Could you check a few things on this drawing? It's one solid part, dimensions in mm from its lowest x, y, z. A direction names the side the tool comes from. Give positions to 0.01 mm unless a question says otherwise; leave off trailing zeros. Write each loop counter-clockwise with the first axis right and the second up, starting at its lowest first coordinate (ties: lowest second). Pieces come first, ordered by that corner, then holes.
1. Suppose I cut it at B-B (y = 170). Please give me the cut outline in (x, z).
2. If I drill on probe 1 along Y at (x, z) = (35, 1.15); probe 2 along Z at (x, y) = (31, 127.5); probe 3 along Y at (x, z) = (13, 27), over which ranges is the centre line in solid material (lowest first)?
3. Suppose I cut it at A-A (x = 35). Please give me the cut outline in (y, z).
4. Thinking about a two-plate mould opening in Z: for the marked faces 4, 5 and 6, which applies, pulls with the +Z half, pulls with the -Z half, needs draft (parallel to the pull), parting line crosses it, or undercut?
5. I'm going to push flat-ended pins straight in: pin 1 (4 mm diameter, centred on x = 69, y = 89.5, fed in from -Z); pin 2 (12.5 mm diameter, centred on x = 31, z = 20.5, fed in from +Y); pin 3 (20 mm diameter, centred on x = 35, y = 170, fed in from +Z). Where does each tip first touch, or does it pass through?
6. Suppose I cut it at D-D (y = 15). Please give me the cut outline in (x, z), and give its area (3 significant figures).
7. Suppose I cut it at C-C (x = 20.5). Please give me the cut outline in (y, z).
8. On a 3-axis mill with a long thin cutter (end or side, diameter ignored), from which of +Z, -Z, +X, -X, +Y, -Y can I reach the whole of each face in a straight line? I mean the marked faces 1, 2 and 3. Say none if no direction works.
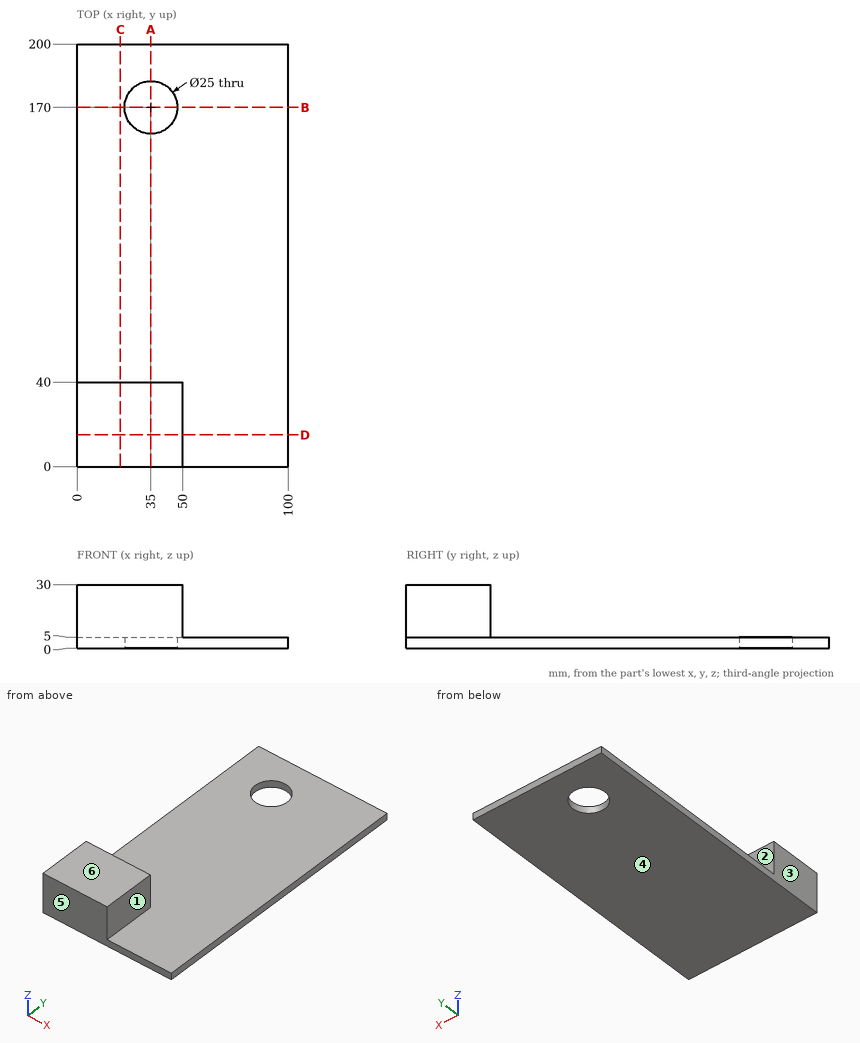
Checks:
1. outline: (0, 0) - (22.5, 0) - (22.5, 5) - (0, 5) - close; (47.5, 0) - (100, 0) - (100, 5) - (47.5, 5) - close
2. probe 1: y = 0 to 157.5, 182.5 to 200
2. probe 2: z = 0 to 5
2. probe 3: y = 0 to 40
3. outline: (0, 0) - (157.5, 0) - (157.5, 5) - (40, 5) - (40, 30) - (0, 30) - close; (182.5, 0) - (200, 0) - (200, 5) - (182.5, 5) - close
4. face 4: pulls with the -Z half
4. face 5: needs draft
4. face 6: pulls with the +Z half
5. pin 1: stops at z = 0
5. pin 2: stops at y = 40
5. pin 3: passes through
6. outline: (0, 0) - (100, 0) - (100, 5) - (50, 5) - (50, 30) - (0, 30) - close
6. area: 1,750 mm2
7. outline: (0, 0) - (200, 0) - (200, 5) - (40, 5) - (40, 30) - (0, 30) - close
8. face 1: +Z, +X, +Y, -Y
8. face 2: +Z, +X, -X, +Y
8. face 3: +Z, -Z, -X, +Y, -Y
